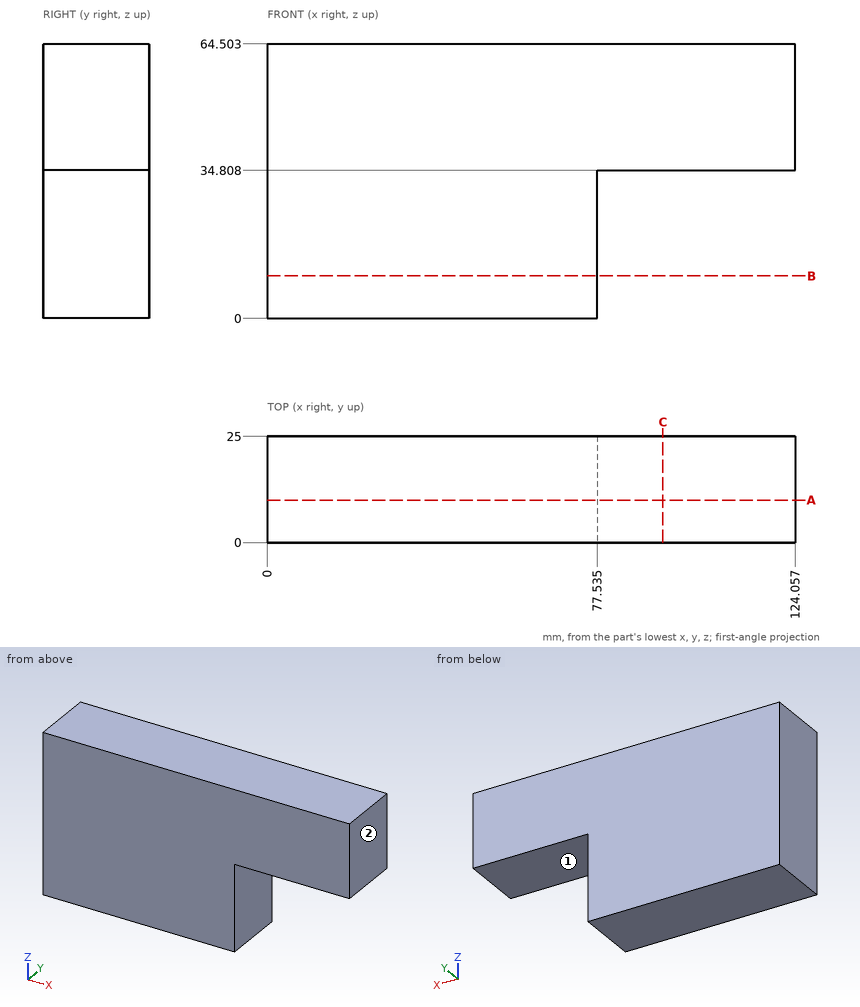
Verification items for this drawing (mm, ordinates from the low corner). A direction names the side the tool comes from. Round coordinates to 2 decimals unless told otherwise and drop trailing zeros. Write each loop counter-clockwise with the first axis right and the second up, starting at its lowest first coordinate (ties: lowest second). Pieces come first, ordered by that corner, then holes. Notation, with made-up numbers: (-9, 85) - (31, 85) arc R34 ccw to (31, 119) - close; hole circle Ø4 at (-7, 66.25). An arc over 180 degrees is marked (long way). Answer as a JSON object with one key per item and string values. Group by question number.
Q1. Section check B-B, the plane z = 10. Enter the section's corners in (x, y) (1 decimal).
Q2. Section check C-C, the plane x = 93. Enter the section's corners in (y, z).
Q3. Go/stop test with flat-tipped pins: pin 1 Ø1.5 at (x, z) = (40.5, 15) entering from -Y; pin 2 Ø1 at (y, z) = (7.5, 14) entering from +X (1 decimal). Record where each tip stops, or that it passes through.
Q4. Section check A-A, the plane y = 10. Enter the section's corners in (x, z) (1 decimal).
Q5. Tool access check on the marked faces 1 and 2. Record the directions out of +Z, -Z, +X, -X, +Y, -Y that give a thin tool (end or side, any length) a straight path to the whole face; none if there is none.
Q6. Thickness scan on line 1 (X direction, y = 18.5, z = 28) (1 decimal); line 2 (Z direction, x = 79, y = 6.75). Record the ranges inside material, lowest first.
Found:
{
 "1": {"outline": "(0, 0) - (77.5, 0) - (77.5, 25) - (0, 25) - close"},
 "2": {"outline": "(0, 34.81) - (25, 34.81) - (25, 64.5) - (0, 64.5) - close"},
 "3": {"pin 1": "stops at y = 0", "pin 2": "stops at x = 77.5"},
 "4": {"outline": "(0, 0) - (77.5, 0) - (77.5, 34.8) - (124.1, 34.8) - (124.1, 64.5) - (0, 64.5) - close"},
 "5": {"face 1": "-Z, +X, +Y, -Y", "face 2": "+Z, -Z, +X, +Y, -Y"},
 "6": {"line 1": "x = 0 to 77.5", "line 2": "z = 34.81 to 64.5"}
}
